Can you work these out from the model? Positions are in its coordinate system, mm. A direction names the side the tool comes from. Coordinates: 2 decimals unless noted, no trailing zeros. Write each loop counter-clockwise with the first axis right and the second up, starting at its lowest first coordinate (ties: lowest second). Pieces come first, ordered by that corner, then holes. Notation, with made-up numbers: (39, 42.5) -> (64, 42.5) arc R30 ccw to (64, 67.5) -> close; hole circle Ø7 at (-31.75, 46.5). An arc over 180 degrees is marked (long way). Use one line per item in the form item = value.
```python
from build123d import *

# Parameters (mm, degrees)
SKETCH_R     = 2.8
PAD_DEPTH    = 3
SKETCH001_R  = 1.45
PAD001_DEPTH = 40
POCKET_DEPTH = 2
CHAMFER_SIZE = 0.25


with BuildPart() as part:
    # Sketch → Pad (new body)
    with BuildSketch(Plane.XY):
        Circle(SKETCH_R)
    extrude(amount=PAD_DEPTH)

    # Sketch001 (on Face3 of Pad) → Pad001 (join)
    with BuildSketch(Plane.XY.offset(3)):
        Circle(SKETCH001_R)
    extrude(amount=PAD001_DEPTH)

    # Sketch002 (on Face2 of Pad001) → Pocket (cut)
    with BuildSketch(Plane(origin=(0, 0, 0), x_dir=(1, 0, 0), z_dir=(0, 0, -1))):
        Polygon((1.259542, 0.814588), (-0.075682, 1.49809), (-1.335225, 0.683502), (-1.259542, -0.814588), (0.075682, -1.49809), (1.335225, -0.683502), align=None)
    extrude(amount=-POCKET_DEPTH, mode=Mode.SUBTRACT)

    # Chamfer
    chamfer_edges = [part.edges().sort_by_distance(p)[0] for p in [
        (-2.8, 0, 3),
        (-2.8, 0, 0),
        (1.297384, -0.065543, 0),
        (0.705454, 1.090796, 0),
        (-0.59193, 1.156339, 0),
        (-1.297384, 0.065543, 0),
        (-0.705454, -1.090796, 0),
        (0.59193, -1.156339, 0),
        (-1.45, 0, 43),
    ]]
    chamfer(chamfer_edges, length=CHAMFER_SIZE)


solid = part.part
```
Q1. Thinking about a two-plate mould opening in Y: for faces 4 (the cylindrical face through (-2.8, 0.1, 1.5)), 5 (the flat face through (2, 0, 0)), 6 (the flat face through (0, 0, 2)), which applies, released by +Y, released by -Y, zero draft, split by the parting line, or undercut?
Return value:
face_4 = split by the parting line
face_5 = zero draft
face_6 = undercut
Q2. If I drill on line 1 (Z direction, x = -2.45, y = -0.25); line 2 (X direction, y = -0.15, z = 21.5); line 3 (Z direction, x = -0.05, y = -0.15), over which ranges is the centre line in solid material (lowest first)? Write a range as from..to.
Return value:
line_1 = 0..3
line_2 = -1.44..1.44
line_3 = 2..43
Q3. Will these pins go through, and if not, where does the flat tip stop? pin 1 (1 mm diameter, centred on y = 0, z = 34, fed in from +X); pin 2 (1 mm diameter, centred on y = 0, z = 10.5, fed in from -X); pin 3 (2 mm diameter, centred on x = 2, z = 32, fed in from +Y).
Return value:
pin_1 = 1.45
pin_2 = -1.45
pin_3 = 1.05
Q4. Suppose I cut it at B-B (y = 0). Write out the boundary of the cut face in (x, z), then the cut area to 3 significant figures.
Return value:
outline = (-2.8, 0.25) -> (-2.55, 0) -> (-1.55, 0) -> (-1.3, 0.25) -> (-1.3, 2) -> (1.3, 2) -> (1.3, 0.25) -> (1.55, 0) -> (2.55, 0) -> (2.8, 0.25) -> (2.8, 2.75) -> (2.55, 3) -> (1.45, 3) -> (1.45, 42.75) -> (1.2, 43) -> (-1.2, 43) -> (-1.45, 42.75) -> (-1.45, 3) -> (-2.55, 3) -> (-2.8, 2.75) -> close
area = 127 mm2
Q5. For faces 1 (the flat face through (0, 0, 43)), 2 (the flat face through (0.76, 1.2, 0.13)), 3 (the flat face through (0, -2, 3)), which set-ups out of +Z, -Z, +X, -X, +Y, -Y let a thin tool reach every point of the face, with its end or its side?
Return value:
face_1 = +Z, +X, -X, +Y, -Y
face_2 = -Z
face_3 = +Z
Q6. Suppose I cut it at A-A (z = 7). Write out the boundary of the cut face in (x, y).
Return value:
outline = circle Ø2.9 at (0, 0)
